Job drawing, mm, ordinate dimensions from the low corner. One solid piece. Coordinates: 2 decimals unless noted, no trailing zeros. Loops run counter-clockwise (first coordinate to the right, second up) from the corner with the lowest first, then second, coordinate; pieces in that order, holes last. Notation, with made-up numbers: (87, 10) - (127, 10) arc R30 cw to (127, 32) - close; hole circle Ø9 at (40.25, 57). An arc over 180 degrees is marked (long way). Use a Markdown table: item, result. Add a question column.
1) Drop flat-ended pins along their axis: P1, Ø8, axis at x = 10, y = 30, coming from the -Z side; P2, Ø2, axis at x = 19, y = 16, coming from the +Z side. Give the stop position or say it passes through.
2) Pull direction Y, two halves, no side cores. Call the marked faces 1, 2 and 3: +Y half, -Y half, draft (parallel to the pull), parting line (faces both ways), or undercut.
3) Band-saw the part on B-B (y = 30). Give the cut face in (x, z).
4) Band-saw the part on A-A (x = 10). Give the cut face in (y, z).
5) Probe probe 1 along Y at (x, z) = (10, 5.5); probe 2 along Z at (x, y) = (2.5, 31); probe 3 along X at (y, z) = (28, 9.25). List the from-to ranges inside material, lowest first. Write a range as [from, to].
6) Band-saw the part on C-C (y = 17). Give the cut face in (x, z).
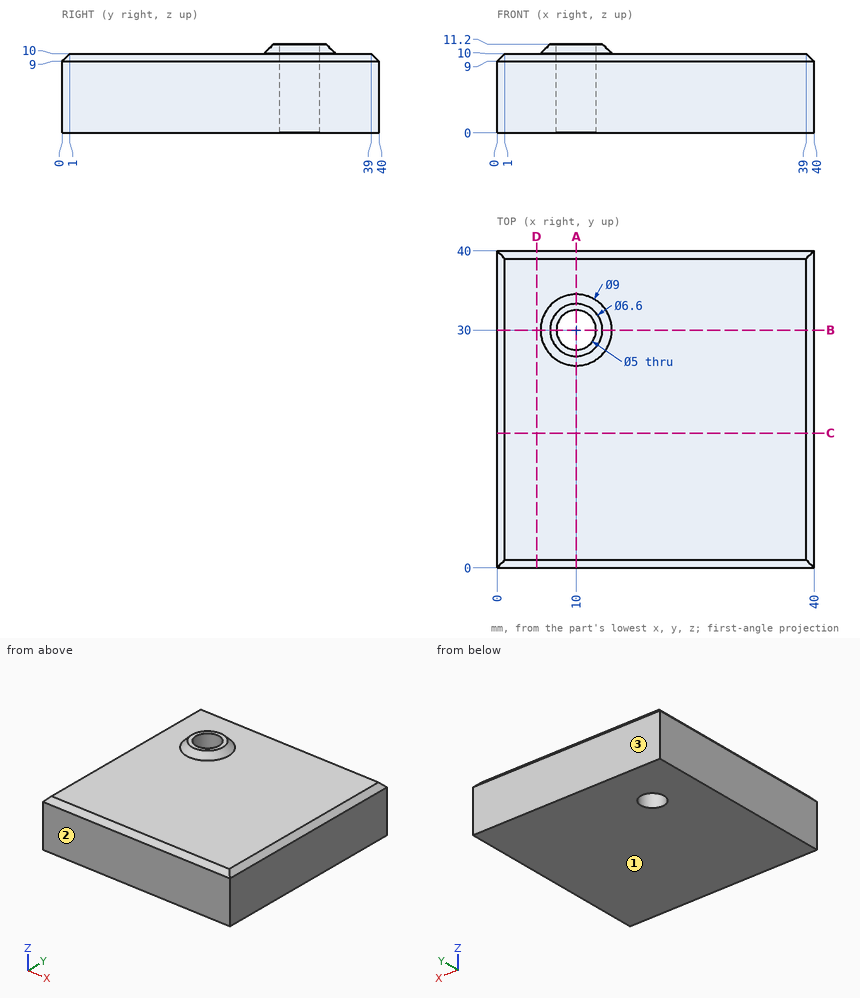
Answer block:
| question | item | result |
|---|---|---|
| 1 | P1 | z = 0 |
| 1 | P2 | z = 10 |
| 2 | face 1 | draft |
| 2 | face 2 | -Y half |
| 2 | face 3 | +Y half |
| 3 | outline | (0, 0) - (7.5, 0) - (7.5, 11.2) - (6.7, 11.2) - (5.5, 10) - (1, 10) - (0, 9) - close; (12.5, 0) - (40, 0) - (40, 9) - (39, 10) - (14.5, 10) - (13.3, 11.2) - (12.5, 11.2) - close |
| 4 | outline | (0, 0) - (27.5, 0) - (27.5, 11.2) - (26.7, 11.2) - (25.5, 10) - (1, 10) - (0, 9) - close; (32.5, 0) - (40, 0) - (40, 9) - (39, 10) - (34.5, 10) - (33.3, 11.2) - (32.5, 11.2) - close |
| 5 | probe 1 | [0, 27.5], [32.5, 40] |
| 5 | probe 2 | [0, 10] |
| 5 | probe 3 | [0.25, 8.5], [11.5, 39.75] |
| 6 | outline | (0, 0) - (40, 0) - (40, 9) - (39, 10) - (1, 10) - (0, 9) - close |
